Answer from the drawing. Dimensions are ordinates in mm from the lowest x, y and z of the part. Round coordinates to 2 decimals unless told otherwise and drop trailing zeros. Order: outer loops, then holes, each group sorted by start corner. A loop starts at its lowest first (then second) coordinate and runs counter-clockwise, first axis right, second up. Notation, with made-up numbers: (7.5, 3) -> (23.5, 3) arc R26 cw to (23.5, 30) -> close; hole circle Ø8 at (-15, 67.25). An arc over 180 degrees is marked (long way). Use a Markdown table: item, result. Add a question column.
Item 1: A cutting plane is placed at D-D, the plane x = 11.43. Determine the outline of the cut face in (y, z) (3 decimals).
Item 2: A cutting plane is placed at A-A, the plane y = 7.25. Determine the outline of the cut face in (x, z).
Item 3: Find the intervals of material crossed by L1, parallel to Y at x = 29.5, z = 2.5; L2, parallel to X at y = 7.75, z = 5.5; L3, parallel to X at y = 7.75, z = 14.25, in increasing order. Write a range as [from, to].
Item 4: A cutting plane is placed at B-B, the plane x = 6.35. Determine the outline of the cut face in (y, z) (3 decimals).
Item 5: A flat-ended cylindrical pin translates along its axis: P1, Ø4, axis at x = 24.5, z = 7, coming from the +Y side. Find the tip coordinate at first contact, or state that the pin passes through.
Item 6: A cutting plane is placed at C-C, the plane z = 15.24. Determine the outline of the cut face in (x, y) (3 decimals), plus the area to 3 significant figures.
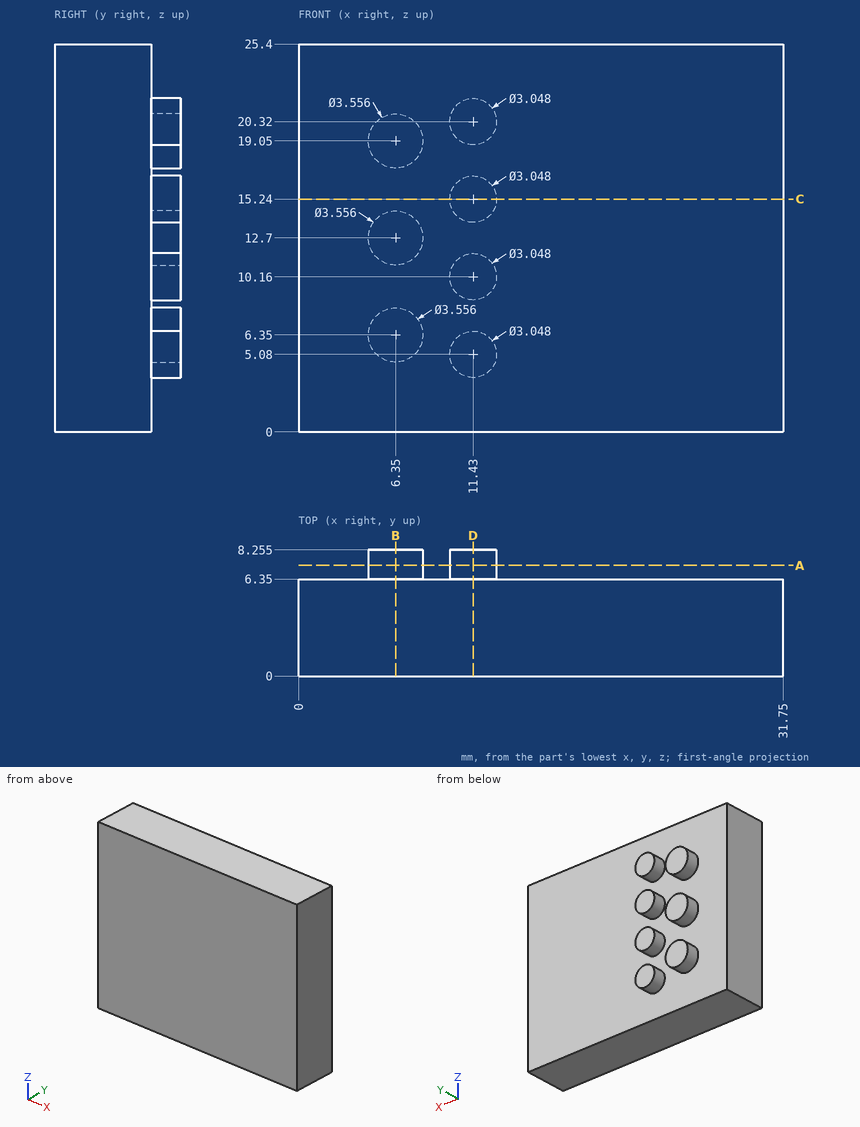
Reported:
| question | item | result |
|---|---|---|
| 1 | outline | (0, 0) -> (6.35, 0) -> (6.35, 3.556) -> (8.255, 3.556) -> (8.255, 6.604) -> (6.35, 6.604) -> (6.35, 8.636) -> (8.255, 8.636) -> (8.255, 11.684) -> (6.35, 11.684) -> (6.35, 13.716) -> (8.255, 13.716) -> (8.255, 16.764) -> (6.35, 16.764) -> (6.35, 18.796) -> (8.255, 18.796) -> (8.255, 21.844) -> (6.35, 21.844) -> (6.35, 25.4) -> (0, 25.4) -> close |
| 2 | outline | circle Ø3.56 at (6.35, 6.35); circle Ø3.56 at (6.35, 12.7); circle Ø3.56 at (6.35, 19.05); circle Ø3.05 at (11.43, 5.08); circle Ø3.05 at (11.43, 10.16); circle Ø3.05 at (11.43, 15.24); circle Ø3.05 at (11.43, 20.32) |
| 3 | L1 | [0, 6.35] |
| 3 | L2 | [4.79, 7.91], [9.97, 12.89] |
| 3 | L3 | [5.48, 7.22], [10.27, 12.59] |
| 4 | outline | (0, 0) -> (6.35, 0) -> (6.35, 4.572) -> (8.255, 4.572) -> (8.255, 8.128) -> (6.35, 8.128) -> (6.35, 10.922) -> (8.255, 10.922) -> (8.255, 14.478) -> (6.35, 14.478) -> (6.35, 17.272) -> (8.255, 17.272) -> (8.255, 20.828) -> (6.35, 20.828) -> (6.35, 25.4) -> (0, 25.4) -> close |
| 5 | P1 | y = 6.35 |
| 6 | outline | (0, 0) -> (31.75, 0) -> (31.75, 6.35) -> (12.954, 6.35) -> (12.954, 8.255) -> (9.906, 8.255) -> (9.906, 6.35) -> (0, 6.35) -> close |
| 6 | area | 207 mm² |
